Design review of the part built by this model. Coordinates are the model's own, in mm. A direction names the side the tool comes from. Coordinates: 2 decimals unless noted, no trailing zeros. Write each loop counter-clockwise with the first axis right and the second up, starting at its lowest first coordinate (ties: lowest second). Pieces come first, ordered by that corner, then holes.
Q1. The part is to be moulded in two halves that separate along Y. For faces 1 (the face through (0, -3, 0)), 2 (the face through (5.49, -7.47, 22.14)), 3 (the face through (0, -1.588, 8)), say which applies: +Y half, -Y half, draft (parallel to the pull), parting line (faces both ways), or undercut.
Q2. To check wall thickness, follow probe 1 along Y at (x, z) = (0, 6.5); probe 2 along Z at (x, y) = (-8.75, 0) (3 decimals); probe 3 along Y at (x, z) = (-3.25, 15). State the ranges of each line that lie inside material, in increasing order.
Q3. Clearance check with flat-ended pins moving along their axes: pin 1 Ø0.6 at (x, z) = (-3, 7.5) entering from +Y; pin 2 Ø1.6 at (x, z) = (3, 9.5) entering from +Y; pin 3 Ø3 at (x, z) = (-3.5, 9.5) entering from -Y. State where each tip first meets the part, or that it passes through.
Q4. Machinability: for faces 4 (the face through (11.025, 7.061, 22.136)), 5 (the face through (1.588, -1, 8)), which of the approach directions +Z, -Z, +X, -X, +Y, -Y give a long, thin tool a straight path to every point of the face, cutting with its end or side? Answer none if there is none.
Q5. Add section D-D, the plane y = -13.5. Give the boundary of the cut face in (x, z) (3 decimals).
Q6. Add section A-A, the plane z = 10.75. Give the boundary of the cut face in (x, y).
from build123d import *

# Parameters (mm, degrees)
F0_R     = 6.35
F1_DEPTH = 15.875
F3_DEPTH = 12.7
F4_SIZE  = 8.88999


# Not quite as in the source:
# - a fillet or chamfer is up to 0.001 mm smaller than in the source, because OpenCascade refuses the exact size


with BuildPart() as f1:
    # F0 (on Top) → F1 (new body)
    with BuildSketch(Plane.XY):
        Circle(F0_R)
        with BuildLine():
            Line((-1.5875, 0), (-3.556, 0))
            ThreePointArc((-3.556, 0), (0, 3.556), (3.556, 0))
            Line((3.556, 0), (1.5875, 0))
            Line((1.5875, 0), (1.5875, -1.5875))
            Line((1.5875, -1.5875), (-1.5875, -1.5875))
            Line((-1.5875, -1.5875), (-1.5875, 0))
        make_face(mode=Mode.SUBTRACT)
    extrude(amount=F1_DEPTH)

    # F2 (on face) → F3 (join)
    with BuildSketch(Plane.XY.offset(15.875)):
        with BuildLine():
            Line((17.2411291662, 7.9984802525), (10.162283151, 13.3764016998))
            Line((10.162283151, 13.3764016998), (-13.1632656924, -17.3265325287))
            ThreePointArc((-13.1632656924, -17.3265325287), (-6.5826089488, -19.0559512579), (-0.7064982299, -15.6256079608))
            Line((-0.7064982299, -15.6256079608), (17.2411291662, 7.9984802525))
        make_face()
        with BuildLine():
            Line((-13.1632656924, -17.3265325287), (10.162283151, 13.3764016998))
            Line((10.162283151, 13.3764016998), (3.0834371358, 18.7543231471))
            Line((3.0834371358, 18.7543231471), (-14.8641902603, -4.8697650662))
            ThreePointArc((-14.8641902603, -4.8697650662), (-16.5936089895, -11.4504218098), (-13.1632656924, -17.3265325287))
        make_face()
    extrude(amount=F3_DEPTH)

    # F4 (size 8.89 in the source; OpenCascade refuses exactly that, so slightly less here)
    f4_edges = [f1.edges().sort_by_distance(p)[0] for p in [
        (3.083437, 18.754323, 22.225),
        (17.241129, 7.99848, 22.225),
    ]]
    chamfer(f4_edges, length=F4_SIZE)


solid = f1.part
Here are the results:
1. face 1: draft
1. face 2: -Y half
1. face 3: undercut
2. probe 1: y = -6.35 to -1.59, 3.56 to 6.35
2. probe 2: z = 15.875 to 28.575
2. probe 3: y = -5.46 to 0, 1.44 to 5.46
3. pin 1: stops at y = 5.75
3. pin 2: stops at y = 5.96
3. pin 3: stops at y = -6.03
4. face 4: +Z, -Z, +X, +Y
4. face 5: -Z
5. outline: (-16.059, 15.875) - (0.908, 15.875) - (0.908, 28.575) - (-16.059, 28.575) - close
6. outline: circle Ø12.7 at (0, 0); hole (-3.56, 0) - (-1.59, 0) - (-1.59, -1.59) - (1.59, -1.59) - (1.59, 0) - (3.56, 0) arc R3.56 ccw to start
